For this review, take the finished solid that the model builds, in its own axes (mm). Face numbers are marked on the shaded views. Give positions to 0.01 mm unless a question says otherwise; leave off trailing zeros. Write each loop counter-clockwise with the first axis right and the second up, starting at its lowest first coordinate (ties: lowest second). Pieces come first, ordered by that corner, then holes.
1) Draft analysis for pull direction X (two halves, no side actions). For the marked faces 1 and 2, state which applies: pulls with the +X half, pulls with the -X half, needs draft (parallel to the pull), parting line crosses it, or undercut.
2) We need section C-C on y = 65. Give the boundary of the cut face in (x, z), and give its area (3 significant figures).
3) We need section D-D on y = 128. Give the boundary of the cut face in (x, z), and give its area (3 significant figures).
4) We need section B-B on y = 90. Give the boundary of the cut face in (x, z), and give its area (3 significant figures).
5) For P1, Ø3, axis at x = 50, y = 200, coming from the +Z side; P2, Ø8, axis at x = 17.5, y = 115, coming from the -Z side; P3, Ø4, axis at x = 29, z = -8.5, coming from the +Y side; P4, Ø3, axis at y = 158, z = -19, coming from the -X side, all flat-tipped, find the tip position at first contact; note any pin that passes through.
6) We need section A-A on z = -15. Give the boundary of the cut face in (x, y), and give its area (3 significant figures).
7) Wall thickness on line 1 along X through (y, z) = (200, 1.2); line 2 along X through (y, z) = (175, 1); line 3 along Y through (x, z) = (32, -9): over which ranges is each line inside the solid? List them lowest first.
Autodesk Fusion 360 part; units mm, degrees
sketch "Sketch1" plane through (0, 0, 0) normal (0, 0, 1) x (1, 0, 0)
  line L0 (5, 5) -> (55, 5)
  line L1 (55, 5) -> (55, 205)
  line L2 (55, 205) -> (5, 205)
  line L3 (5, 205) -> (5, 5)
  line L4 (5, 205) -> (5, 200)
  line L5 (5, 200) -> (10, 200)
  circle A0 centre (10, 200) radius 2.5
  line L6 (5, 5) -> (5, 10)
  line L7 (5, 10) -> (10, 10)
  circle A1 centre (10, 10) radius 2.5
  line L8 (30, 205) -> (30, 5)
  circle A2 centre (50, 200) radius 2.5
  circle A3 centre (50, 10) radius 2.5
  dimension "d1" = 50
  dimension "d2" = 200
  dimension "d3" = 5
  dimension "d4" = 5
extrude "Extrude1" add sketch "Sketch1" along normal blind 3
sketch "Sketch2" plane through (0, 0, 3) normal (0, 0, 1) x (1, 0, 0)
  circle A0 centre (10, 200) radius 2.5
  circle A1 centre (50, 200) radius 2.5
  circle A2 centre (10, 10) radius 2.5
  circle A3 centre (50, 10) radius 2.5
  line L0 (55, 5) -> (55, 205)
  line L1 (55, 205) -> (5, 205)
  line L2 (5, 205) -> (5, 5)
  line L3 (5, 5) -> (55, 5)
  line L4 (5, 205) -> (17.5, 205)
  line L5 (17.5, 205) -> (17.5, 5)
  line L6 (55, 205) -> (42.5, 205)
  line L7 (42.5, 205) -> (42.5, 5)
  line L8 (30, 205) -> (30, 5)
  line L9 (5, 205) -> (5, 185)
  line L10 (5, 5) -> (5, 25)
  line L11 (5, 25) -> (55, 25)
  line L12 (5, 185) -> (55, 185)
  line L13 (17.5, 185) -> (17.5, 175)
  circle A4 centre (17.5, 175) radius 1.75
  line L14 (17.5, 25) -> (17.5, 45)
  circle A5 centre (17.5, 45) radius 4.75
  line L15 (17.5, 45) -> (17.5, 65)
  circle A6 centre (17.5, 65) radius 4.75
  line L16 (17.5, 175) -> (17.5, 155)
  circle A7 centre (17.5, 155) radius 3.5
  line L17 (17.5, 155) -> (17.5, 135)
  circle A8 centre (17.5, 135) radius 3.5
  line L18 (17.5, 135) -> (17.5, 115)
  circle A9 centre (17.5, 115) radius 3
  line L19 (17.5, 115) -> (17.5, 90)
  circle A10 centre (17.5, 90) radius 8
  circle A11 centre (42.5, 175) radius 1.75
  circle A12 centre (42.5, 155) radius 3.5
  circle A13 centre (42.5, 135) radius 3.5
  circle A14 centre (42.5, 115) radius 3
  circle A15 centre (42.5, 90) radius 8
  circle A16 centre (42.5, 65) radius 4.75
  circle A17 centre (42.5, 45) radius 4.75
  dimension "d7" = 12.5
  dimension "d8" = 200
  dimension "d9" = 12.5
  dimension "d10" = 20
  dimension "d11" = 20
  dimension "d12" = 10
  dimension "d13" = 3.5
  dimension "d14" = 20
  dimension "d15" = 9.5
  dimension "d16" = 20
  dimension "d17" = 9.5
  dimension "d18" = 20
  dimension "d19" = 7
  dimension "d20" = 20
  dimension "d21" = 7
  dimension "d22" = 20
  dimension "d23" = 6
  dimension "d24" = 25
  dimension "d25" = 16
extrude "Extrude2" cut sketch "Sketch2" against normal blind 3 contours L7 A17 | L7 A17 | L7 A11 | L7 A11 | L7 A16 | L7 A16 | L5 L14 A5 L15 | L5 L14 A5 L15 | L7 A12 | L7 A12 | L5 L13 A4 L16 | L5 L13 A4 L16 | L7 A15 | L7 A15 | L5 L15 A6 | L5 L15 A6 | L7 A13 | L7 A13 | L5 L16 A7 L17 | L5 L16 A7 L17 | L7 A14 | L7 A14 | L5 L19 A10 | L5 L19 A10 | L5 L17 A8 L18 | L5 L17 A8 L18 | L5 L18 A9 L19 | L5 L18 A9 L19
sketch "Sketch3" plane through (0, 0, 0) normal (0, 0, -1) x (-1, 0, 0)
  circle A0 centre (-42.5, 135) radius 3.5
  circle A1 centre (-42.5, 45) radius 4.75
  circle A2 centre (-17.5, 115) radius 3
  circle A3 centre (-17.5, 155) radius 3.5
  circle A4 centre (-17.5, 90) radius 8
  circle A5 centre (-42.5, 65) radius 4.75
  circle A6 centre (-42.5, 155) radius 3.5
  circle A7 centre (-42.5, 115) radius 3
  circle A8 centre (-17.5, 45) radius 4.75
  circle A9 centre (-17.5, 135) radius 3.5
  circle A10 centre (-17.5, 175) radius 1.75
  circle A11 centre (-17.5, 65) radius 4.75
  circle A12 centre (-42.5, 90) radius 8
  circle A13 centre (-42.5, 175) radius 1.75
  circle A14 centre (-10, 200) radius 2.5
  circle A15 centre (-50, 200) radius 2.5
  circle A16 centre (-10, 10) radius 2.5
  circle A17 centre (-50, 10) radius 2.5
  line L0 (-55, 205) -> (-55, 5)
  line L1 (-55, 5) -> (-5, 5)
  line L2 (-5, 5) -> (-5, 205)
  line L3 (-5, 205) -> (-55, 205)
  line L4 (-55, 205) -> (-55, 185)
  line L5 (-55, 185) -> (-52, 185)
  line L6 (-52, 185) -> (-52, 25)
  line L7 (-52, 25) -> (-55, 25)
  line L8 (-55, 25) -> (-55, 185)
  line L9 (-30, 205) -> (-30, 5)
  line L10 (-5, 25) -> (-5, 185)
  line L11 (-8, 185) -> (-8, 25)
  line L12 (-8, 25) -> (-5, 25)
  line L13 (-5, 185) -> (-8, 185)
  dimension "d28" = 20
  dimension "d29" = 3
  dimension "d30" = 160
extrude "Extrude3" add sketch "Sketch3" along normal blind 5 contours L0 L5 L6 L7 L8 | L2 L10 L11 L12 L13
chamfer "Chamfer1" distance 5 angle 45 4 edges at (6.5, 25, -5) (53.5, 25, -5) (6.5, 185, -5) (53.5, 185, -5)
sketch "Sketch4" plane through (0, 0, 0) normal (1, 0, 0) x (0, 0, -1)
sketch "Sketch5" plane through (0, 0, 0) normal (0, 0, -1) x (-1, 0, 0)
  circle A0 centre (-42.5, 135) radius 3.5
  circle A1 centre (-42.5, 45) radius 4.75
  circle A2 centre (-17.5, 115) radius 3
  circle A3 centre (-17.5, 155) radius 3.5
  circle A4 centre (-17.5, 90) radius 8
  circle A5 centre (-42.5, 65) radius 4.75
  circle A6 centre (-42.5, 155) radius 3.5
  circle A7 centre (-42.5, 115) radius 3
  circle A8 centre (-17.5, 45) radius 4.75
  circle A9 centre (-17.5, 135) radius 3.5
  circle A10 centre (-17.5, 175) radius 1.75
  circle A11 centre (-17.5, 65) radius 4.75
  circle A12 centre (-42.5, 90) radius 8
  circle A13 centre (-42.5, 175) radius 1.75
  circle A14 centre (-10, 200) radius 2.5
  circle A15 centre (-50, 200) radius 2.5
  circle A16 centre (-10, 10) radius 2.5
  circle A17 centre (-50, 10) radius 2.5
  line L0 (-5, 25) -> (-8, 25)
  line L1 (-8, 25) -> (-8, 185)
  line L2 (-8, 185) -> (-5, 185)
  line L3 (-5, 185) -> (-5, 205)
  line L4 (-5, 205) -> (-55, 205)
  line L5 (-55, 205) -> (-55, 185)
  line L6 (-55, 185) -> (-52, 185)
  line L7 (-52, 185) -> (-52, 25)
  line L8 (-52, 25) -> (-55, 25)
  line L9 (-55, 25) -> (-55, 5)
  line L10 (-55, 5) -> (-5, 5)
  line L11 (-5, 5) -> (-5, 25)
  line L12 (-30, 205) -> (-30, 5)
  line L13 (-30, 205) -> (-30, 165)
  line L14 (-30, 5) -> (-30, 50)
  line L15 (-30, 165) -> (-27.5, 165)
  line L16 (-27.5, 165) -> (-27.5, 155)
  line L17 (-27.5, 155) -> (-30, 155)
  line L18 (-30, 155) -> (-30, 165)
  line L19 (-30, 165) -> (-32.5, 165)
  line L20 (-32.5, 165) -> (-32.5, 155)
  line L21 (-32.5, 155) -> (-30, 155)
  line L22 (-30, 155) -> (-30, 165)
  line L23 (-52, 105) -> (-8, 105)
  line L24 (-27.5, 55) -> (-30, 55)
  line L25 (-27.5, 45) -> (-27.5, 55)
  line L26 (-30, 45) -> (-27.5, 45)
  line L27 (-30, 45) -> (-32.5, 45)
  line L28 (-32.5, 45) -> (-32.5, 55)
  line L29 (-32.5, 55) -> (-30, 55)
  dimension "d34" = 40
  dimension "d35" = 45
  dimension "d36" = 2.5
  dimension "d37" = 10
extrude "Extrude4" add sketch "Sketch5" along normal blind 30 contours L12 L14 L27 L28 L29 | L12 L14 L24 L25 L26
extrude "Extrude5" add sketch "Sketch5" along normal blind 30 contours L12 L18 L19 L20 L21 L22 | L12 L15 L16 L17 L18 L22
fillet "Fillet1" radius 5 4 edges at (30, 155, -30) (30, 165, -30) (30, 55, -30) (30, 45, -30)
sketch "Sketch6" plane through (27.5, 0, 0) normal (-1, 0, 0) x (0, 0, 1)
  arc A0 (-25, 165) -> (-25, 155) centre (-25, 160) ccw
  line L0 (-25, 155) -> (0, 155)
  line L1 (0, 155) -> (0, 165)
  line L2 (0, 165) -> (-25, 165)
  line L3 (-30, 160) -> (-25, 160)
  line L4 (-30, 50) -> (-25, 50)
  circle A1 centre (-25, 50) radius 1.75
  circle A2 centre (-25, 160) radius 1.75
  dimension "d43" = 3.5
  dimension "d44" = 3.5
extrude "Extrude6" cut sketch "Sketch6" against normal blind 5 contours A2 | A1
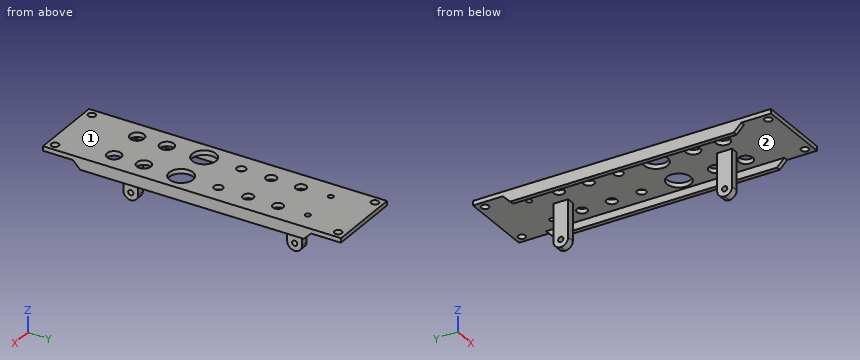
Results list:
1. face 1: needs draft
1. face 2: undercut
2. outline: (5, -5) - (8, -5) - (8, 0) - (12.75, 0) - (12.75, 3) - (5, 3) - close; (22.25, 0) - (37.75, 0) - (37.75, 3) - (22.25, 3) - close; (47.25, 0) - (52, 0) - (52, -5) - (55, -5) - (55, 3) - (47.25, 3) - close
2. area: 123 mm2
3. outline: (5, -5) - (8, -5) - (8, 0) - (52, 0) - (52, -5) - (55, -5) - (55, 3) - (5, 3) - close
3. area: 180 mm2
4. outline: (5, -5) - (8, -5) - (8, 0) - (9.5, 0) - (9.5, 3) - (5, 3) - close; (25.5, 0) - (34.5, 0) - (34.5, 3) - (25.5, 3) - close; (50.5, 0) - (52, 0) - (52, -5) - (55, -5) - (55, 3) - (50.5, 3) - close
4. area: 84.0 mm2
5. P1: passes through
5. P2: stops at z = 0
5. P3: stops at y = 165
5. P4: stops at x = 27.5
6. outline: (27.5, 45) - (32.5, 45) - (32.5, 55) - (27.5, 55) - close; (27.5, 155) - (32.5, 155) - (32.5, 165) - (27.5, 165) - close
6. area: 100 mm2
7. line 1: x = 5 to 7.5, 12.5 to 47.5, 52.5 to 55
7. line 2: x = 5 to 15.75, 19.25 to 40.75, 44.25 to 55
7. line 3: y = 45 to 55, 155 to 165
